Input: part model. Units: mm. Frame: model coordinates. Coordinates: 2 decimals unless noted, no trailing zeros. Order: outer loops, then holes, each group sorted by start corner. A loop starts at its lowest first (then second) coordinate and runs counter-clockwise, first axis right, second up. Notation, with made-up numbers: (51.5, -14.75) -> (96.5, -14.75) arc R33 cw to (96.5, 20.25) -> close; hole circle Ø1 at (76, 63.25). An arc over 180 degrees is marked (long way). Use one line per item in the form item = value. Start each with the question number.
1) Section query C-C on y = -4. Output: boundary loops of the cut face in (x, z).
2) Section query D-D on y = -29. Output: boundary loops of the cut face in (x, z), then the cut area to 3 significant figures.
3) Section query B-B on y = -15.5. Output: boundary loops of the cut face in (x, z).
4) Pin query (flat end, axial travel): pin 1 (8 mm diameter, centred on x = 52, y = -10.5, fed in from -Z). Return the tip coordinate at first contact, or that it passes through.
5) Ray query, line 1 along X through (y, z) = (-16.5, 0.2); line 2 along Y through (x, z) = (48, 0.5); line 3 along X through (y, z) = (-1.5, 0.35). Return the intervals inside material, ascending.
from build123d import *

# Parameters (mm, degrees)
F1_DEPTH = 0.762


with BuildPart() as f1:
    # F0 (on Top) → F1 (new body)
    with BuildSketch(Plane.XY):
        with BuildLine():
            Line((41.4909, 0), (10.0076, 0))
            Line((10.0076, 0), (1.041983, -4.915161))
            Line((1.041983, -4.915161), (0, -5.4864))
            Line((0, -5.4864), (0, -6.674694))
            Line((0, -6.674694), (0, -27.5082))
            Line((0, -27.5082), (10.0076, -32.9946))
            Line((10.0076, -32.9946), (41.4909, -32.9946))
            ThreePointArc((41.4909, -32.9946), (57.9882, -16.4973), (41.4909, 0))
        make_face()
        with BuildLine():
            Line((18.986508, -18.042571), (18.999208, -14.956523))
            ThreePointArc((18.999208, -14.956523), (19.290783, -14.2587), (19.9898, -13.97))
            ThreePointArc((19.9898, -13.97), (20.688817, -14.2587), (20.980392, -14.956523))
            Line((20.980392, -14.956523), (20.993092, -18.042571))
            ThreePointArc((20.993092, -18.042571), (20.700698, -18.754679), (19.9898, -19.05))
            ThreePointArc((19.9898, -19.05), (19.278902, -18.754679), (18.986508, -18.042571))
        make_face(mode=Mode.SUBTRACT)
    extrude(amount=F1_DEPTH)


solid = f1.part
Answers below:
q1.outline = (2.71, 0) -> (52.26, 0) -> (52.26, 0.76) -> (2.71, 0.76) -> close
q2.outline = (2.72, 0) -> (52.25, 0) -> (52.25, 0.76) -> (2.72, 0.76) -> close
q2.area = 37.7 mm^2
q3.outline = (0, 0) -> (19, 0) -> (19, 0.76) -> (0, 0.76) -> close; (20.98, 0) -> (57.96, 0) -> (57.96, 0.76) -> (20.98, 0.76) -> close
q4.pin_1 = 0
q5.line_1 = 0 to 18.99, 20.99 to 57.99
q5.line_2 = -31.66 to -1.34
q5.line_3 = 7.27 to 48.36
